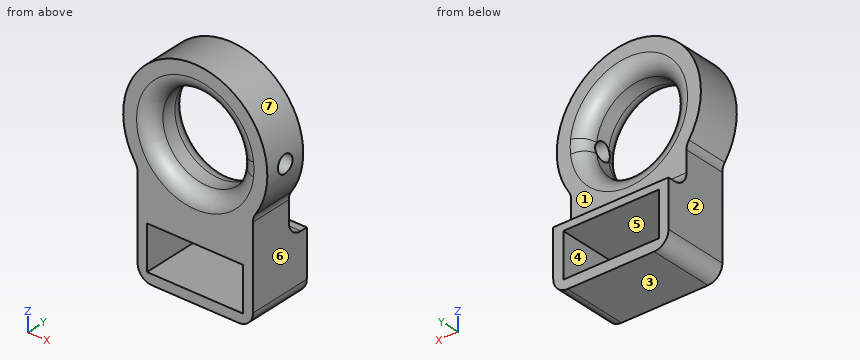
Autodesk Inventor part; units mm, degrees
ref_plane "Plano de trabajo6" through (0, 0, -10) normal (0, 0, 1) x (1, 0, 0)
ref_plane "Plano de trabajo5" through (10, 0, 0) normal (1, 0, 0) x (0, 1, 0)
ref_plane "YZ Plane" through (0, 0, 0) normal (1, 0, 0) x (0, 1, 0)
sketch "Boceto1" plane through (0, 0, 0) normal (0, 1, 0) x (-1, 0, 0)
  circle A0 centre (0, 0) radius 10
  dimension "d0" = 20
extrude "Extrusión1" add sketch "Boceto1" along normal blind 6
ref_plane "Plano de trabajo6" through (0, 0, -10) normal (0, 0, 1) x (1, 0, 0)
sketch "Boceto3" plane through (0, 0, -10) normal (0, 0, 1) x (1, 0, 0)
  line L0 (10, 0) -> (-10, 0)
  line L1 (8, 0) -> (8, 10)
  line L2 (10, 10) -> (-10, 10)
  line L3 (8, 10) -> (-8, 10)
  line L4 (-8, 10) -> (-8, 0)
  line L5 (-8, 0) -> (8, 0)
  point P0 (0, 0)
  dimension "d10" = 8
  dimension "d11" = 10
  dimension "d12" = 16
extrude "Extrusión2" add sketch "Boceto3" along normal blind 5 and the other way blind 7
sketch "Boceto4" plane through (0, 6, 0) normal (0, 1, 0) x (1, 0, 0)
  line L0 (-8, 17) -> (8, 17)
  line L1 (-6.7, 15.6) -> (6.6, 15.6)
  line L2 (6.6, 15.6) -> (6.6, 9.5)
  line L3 (6.6, 9.5) -> (-6.7, 9.5)
  line L4 (-6.7, 9.5) -> (-6.7, 15.6)
  line L5 (-6.6, 18.5) -> (6.6, 12.5) construction
  line L6 (6.6, 18.5) -> (-6.6, 12.5) construction
  point P0 (0, 0)
  dimension "d19" = 13.3
  dimension "d20" = 6.1
extrude "Extrusión3" cut sketch "Boceto4" against normal blind 10
sketch "Boceto5" plane through (0, 6, 0) normal (0, 1, 0) x (1, 0, 0)
  arc A0 (-8, 6) -> (8, 6) centre (0, 0) ccw
hole "Agujero2" at (0, 6, 0) direction (0, -1, 0) diameter 12.3 end through all
ref_plane "Plano de trabajo5" through (10, 0, 0) normal (1, 0, 0) x (0, 1, 0)
sketch "Boceto6" plane through (10, 0, 0) normal (1, 0, 0) x (0, 1, 0)
  line L0 (0, 0) -> (3, 0)
  dimension "d32" = 3
hole "Agujero3" at (10, 3, 0) direction (-1, 0, 0) diameter 2.459 depth 5
sketch "Boceto7" plane through (0, 0, -5) normal (0, 0, 1) x (1, 0, 0)
  line L0 (-8, 6) -> (-8.3333, 6)
  line L1 (8, 10) -> (-8, 10)
  line L2 (-8, 10) -> (-8, 6)
  line L3 (-8, 6) -> (8, 6)
  line L4 (8, 6) -> (8, 10)
  point P0 (0, 0)
extrude "Extrusión4" cut sketch "Boceto7" against normal blind 17
fillet "Empalme4" radius 2 2 edges at (0, 6, -6.15) (0, 0, -6.15)
sketch "Boceto8" plane through (0, 6, 0) normal (0, 1, 0) x (1, 0, 0)
  line L0 (-8, 6) -> (-8, 17)
  line L1 (-8, 17) -> (8, 17)
  line L2 (8, 17) -> (8, 8.5)
  line L3 (8, 8.5) -> (-8, 8.5)
  line L4 (-8, 8.5) -> (-8, 17)
  point P0 (0, 0)
  dimension "d45" = 16
  dimension "d46" = 8.5
extrude "Extrusión5" add sketch "Boceto8" along normal blind 3
sketch "Boceto9" plane through (0, 0, -17) normal (0, 0, -1) x (-1, 0, 0)
  line L0 (-8, 9) -> (-8, 0)
  line L1 (8, 0) -> (8, 9)
  line L2 (-8, 9) -> (8, 9)
  line L3 (8, 9) -> (8, 0)
  line L4 (8, 0) -> (-8, 0)
  line L5 (-8, 0) -> (-8, 9)
  point P0 (0, 0)
extrude "Extrusión6" add sketch "Boceto9" along normal blind 3
sketch "Boceto10" plane through (6.6, 0, -9.5) normal (0, 0, -1) x (-1, 0, 0)
  line L0 (0, 6) -> (0, 0)
  line L1 (13.3, 6) -> (13.3, 0)
  line L2 (0, 6) -> (13.3, 6)
  line L3 (13.3, 6) -> (13.3, 0)
  line L4 (13.3, 0) -> (0, 0)
  line L5 (0, 0) -> (0, 6)
  point P0 (6.6, 0)
extrude "Extrusión7" add sketch "Boceto10" along normal blind 3
sketch "Boceto11" plane through (-6.7, 0, -15.6) normal (0, 0, 1) x (1, 0, 0)
  line L0 (13.3, 6) -> (0, 6)
  line L1 (13.3, 0) -> (0, 0)
  line L2 (0, 6) -> (13.3, 6)
  line L3 (13.3, 6) -> (13.3, 0)
  line L4 (13.3, 0) -> (0, 0)
  line L5 (0, 0) -> (0, 6)
  point P0 (6.7, 0)
extrude "Extrusión8" cut sketch "Boceto11" against normal blind 3
sketch "Boceto12" plane through (-8, 6, -8.5) normal (0, 0, 1) x (1, 0, 0)
  line L0 (16, 0) -> (16, 3)
  line L1 (16, 3) -> (0, 3)
  line L2 (0, 3) -> (0, 0)
  line L3 (0, 0) -> (16, 0)
  line L4 (16, 0) -> (16, 3)
  point P0 (8, -6)
extrude "Extrusión9" cut sketch "Boceto12" against normal blind 3
sketch "Boceto13" plane through (0, 6, 0) normal (0, -1, 0) x (1, 0, 0)
  line L0 (6.6, -12.5) -> (-6.7, -12.5)
  line L1 (-6.7, -12.5) -> (-6.7, -18.6)
  line L2 (6.6, -12.5) -> (-6.7, -12.5)
  line L3 (-6.7, -12.5) -> (-6.7, -18.6)
  line L4 (-6.7, -18.6) -> (6.6, -18.6)
  line L5 (6.6, -18.6) -> (6.6, -12.5)
  point P0 (0, 0)
extrude "Extrusión10" cut sketch "Boceto13" against normal blind 3
fillet "Empalme5" radius 2 4 edges at (8, 4.5, -20) (-8, 4.5, -20) (-8, 3, -6) (8, 3, -6)
fillet "Empalme6" radius 2 1 edges at (0, 6, -11.5)
properties part number "Final Carrera Y0"
Could you check a few things on this model? Use its own coordinates, in mm. Face numbers are marked on the shaded views. A direction names the side the tool comes from. Round coordinates to 2 decimals unless told otherwise and drop trailing zeros. Order: outer loops, then holes, each group sorted by start corner. A loop starts at its lowest first (then second) coordinate and runs counter-clockwise, first axis right, second up.
(1) Imagine slicing it at A-A (z = -16.5). Write out the boundary of the cut face in (x, y).
Response values:
outline: (-8, 0) - (-6.7, 0) - (-6.7, 9) - (-8, 9) - close; (6.6, 0) - (8, 0) - (8, 9) - (6.6, 9) - close
(2) Please list where these lines run through material, in increasing order: line 1 along Z through (x, y) = (0, 2.6); line 2 along Y through (x, z) = (8.9, 0); line 3 along Z through (x, y) = (-2, 4.5).
Response values:
line 1: z = -20 to -18.6, -12.5 to -6.15, 6.15 to 10
line 2: y = 0 to 1.77, 4.23 to 6
line 3: z = -20 to -18.6, -12.5 to -5.88, 5.88 to 9.8
(3) I'm going to push flat-ended pins straight in: pin 1 (2.5 mm diameter, centred on y = 5.5, z = -12.5, fed in from -X); pin 2 (6 mm diameter, centred on x = 4.5, z = 3.5, fed in from +Y); pin 3 (5 mm diameter, centred on y = 5.5, z = -16.5, fed in from +X); pin 4 (4 mm diameter, centred on x = 3.5, z = -1, fed in from +Y). Where does each tip first touch, or does it pass through?
Response values:
pin 1: stops at x = -8
pin 2: stops at y = 6
pin 3: stops at x = 8
pin 4: passes through
(4) Imagine slicing it at B-B (z = 0). Count the separate pieces of the cut face and the enclosed holes in it, plus the area to 3 significant figures.
Response values:
separate pieces: 3
enclosed holes: 0
area: 33.3 mm2
(5) If we mould it in two halves opening along Z, with no side actions, what happens to the marked faces 5, 6 and 7? For each: released by +Z, released by -Z, zero draft, split by the parting line, or undercut.
Response values:
face 5: undercut
face 6: zero draft
face 7: split by the parting line
(6) Which directions (+Z, -Z, +X, -X, +Y, -Y) give clear straight access to the entire face, cutting with the end or side of a thin tool? Please do the marked faces 1, 2, 3 and 4.
Response values:
face 1: +Z, +X, -X, +Y
face 2: -Z, -X, +Y, -Y
face 3: -Z, +X, -X, +Y, -Y
face 4: +Y, -Y
(7) Imagine slicing it at D-D (y = 3). Write out the boundary of the cut face in (x, z), plus the area to 3 significant figures.
Response values:
outline: (-8.33, -5.53) arc R2 cw to (-8, -6.63) - (-8, -18) arc R2 ccw to (-6, -20) - (6, -20) arc R2 ccw to (8, -18) - (8, -6.63) arc R2 cw to (8.33, -5.53) arc R10 ccw to (9.92, -1.23) - (6.03, -1.23) arc R6.15 cw (long way) to (6.03, 1.23) - (9.92, 1.23) arc R10 ccw (long way) to start; hole (-6.7, -18.6) - (6.6, -18.6) - (6.6, -12.5) - (-6.7, -12.5) - close
area: 282 mm2
